```python
from build123d import *

# Parameters (mm, degrees)
SKETCH_1_R      = 1.55
SKETCH_1_W      = 22
SKETCH_1_H      = 14.8
EXTRUDE_1_DEPTH = 4
FILLET_4_R      = 3
FILLET_2_R      = 1.5


with BuildPart() as part:
    # 草图1 → 凸台-拉伸1 (new body)
    with BuildSketch(Plane.XY):
        Polygon((19, 14.5), (19, 13.5), (-18, 13.5), (-19, 13.5), (-19, -13.5), (14, -13.5), (19, -24.5), (55, -24.5), (55, 14.5), align=None)
        with BuildLine():
            ThreePointArc((-18, -9.390512484), (-18.05, -9), (-18, -8.609487516))
            ThreePointArc((-18, -8.609487516), (-14.95, -9), (-18, -9.390512484))
        make_face(mode=Mode.SUBTRACT)
        with Locations((16.5, -9)):
            Circle(SKETCH_1_R, mode=Mode.SUBTRACT)
        with BuildLine():
            ThreePointArc((31.95, -17.4), (33, -16.35), (34.05, -17.4))
            Line((34.05, -17.4), (34.05, -20.45))
            ThreePointArc((34.05, -20.45), (33, -21.5), (31.95, -20.45))
            Line((31.95, -20.45), (27.95, -20.45))
            ThreePointArc((27.95, -20.45), (26.9, -21.5), (25.85, -20.45))
            Line((25.85, -20.45), (25.85, -17.4))
            ThreePointArc((25.85, -17.4), (26.9, -16.35), (27.95, -17.4))
            Line((27.95, -17.4), (31.95, -17.4))
        make_face(mode=Mode.SUBTRACT)
        with BuildLine():
            ThreePointArc((47.95, -17.4), (49, -16.35), (50.05, -17.4))
            Line((50.05, -17.4), (50.05, -20.45))
            ThreePointArc((50.05, -20.45), (49, -21.5), (47.95, -20.45))
            Line((47.95, -20.45), (43.95, -20.45))
            ThreePointArc((43.95, -20.45), (42.9, -21.5), (41.85, -20.45))
            Line((41.85, -20.45), (41.85, -17.4))
            ThreePointArc((41.85, -17.4), (42.9, -16.35), (43.95, -17.4))
            Line((43.95, -17.4), (47.95, -17.4))
        make_face(mode=Mode.SUBTRACT)
        with Locations((22, -12.5)):
            Circle(SKETCH_1_R, mode=Mode.SUBTRACT)
        with BuildLine():
            ThreePointArc((-11.045643943, -6.5), (-11.868221008, -5.185996413), (-13, -4.126602828))
            Line((-13, -4.126602828), (-13, -1.25))
            Line((-13, -1.25), (-2, -1.25))
            Line((-2, -1.25), (-2, -6.5))
            Line((-2, -6.5), (-11.045643943, -6.5))
        make_face(mode=Mode.SUBTRACT)
        with BuildLine():
            Line((-11.045643943, 6.5), (-2, 6.5))
            Line((-2, 6.5), (-2, 1.25))
            Line((-2, 1.25), (-13, 1.25))
            Line((-13, 1.25), (-13, 4.126602828))
            ThreePointArc((-13, 4.126602828), (-11.868221008, 5.185996413), (-11.045643943, 6.5))
        make_face(mode=Mode.SUBTRACT)
        with BuildLine():
            ThreePointArc((13, -4.126602828), (11.868221008, -5.185996413), (11.045643943, -6.5))
            Line((11.045643943, -6.5), (2, -6.5))
            Line((2, -6.5), (2, -1.25))
            Line((2, -1.25), (13, -1.25))
            Line((13, -1.25), (13, -4.126602828))
        make_face(mode=Mode.SUBTRACT)
        with BuildLine():
            Line((2, 6.5), (11.045643943, 6.5))
            ThreePointArc((11.045643943, 6.5), (11.868221008, 5.185996413), (13, 4.126602828))
            Line((13, 4.126602828), (13, 1.25))
            Line((13, 1.25), (2, 1.25))
            Line((2, 1.25), (2, 6.5))
        make_face(mode=Mode.SUBTRACT)
        with BuildLine():
            ThreePointArc((-18, 8.609487516), (-18.05, 9), (-18, 9.390512484))
            ThreePointArc((-18, 9.390512484), (-14.95, 9), (-18, 8.609487516))
        make_face(mode=Mode.SUBTRACT)
        with Locations((16.5, 9)):
            Circle(SKETCH_1_R, mode=Mode.SUBTRACT)
        with Locations((22, 2.5)):
            Circle(SKETCH_1_R, mode=Mode.SUBTRACT)
        with Locations((37, -5)):
            Rectangle(SKETCH_1_W, SKETCH_1_H, mode=Mode.SUBTRACT)
        with Locations((52, -5)):
            Circle(SKETCH_1_R, mode=Mode.SUBTRACT)
        with BuildLine():
            ThreePointArc((27.95, 7.4), (26.9, 6.35), (25.85, 7.4))
            Line((25.85, 7.4), (25.85, 10.45))
            ThreePointArc((25.85, 10.45), (26.9, 11.5), (27.95, 10.45))
            Line((27.95, 10.45), (31.95, 10.45))
            ThreePointArc((31.95, 10.45), (33, 11.5), (34.05, 10.45))
            Line((34.05, 10.45), (34.05, 7.4))
            ThreePointArc((34.05, 7.4), (33, 6.35), (31.95, 7.4))
            Line((31.95, 7.4), (27.95, 7.4))
        make_face(mode=Mode.SUBTRACT)
        with BuildLine():
            ThreePointArc((43.95, 7.4), (42.9, 6.35), (41.85, 7.4))
            Line((41.85, 7.4), (41.85, 10.45))
            ThreePointArc((41.85, 10.45), (42.9, 11.5), (43.95, 10.45))
            Line((43.95, 10.45), (47.95, 10.45))
            ThreePointArc((47.95, 10.45), (49, 11.5), (50.05, 10.45))
            Line((50.05, 10.45), (50.05, 7.4))
            ThreePointArc((50.05, 7.4), (49, 6.35), (47.95, 7.4))
            Line((47.95, 7.4), (43.95, 7.4))
        make_face(mode=Mode.SUBTRACT)
    extrude(amount=EXTRUDE_1_DEPTH)

    # 圆角4
    fillet_4_edges = [part.edges().sort_by_distance(p)[0] for p in [
        (48, -12.4, 2),
        (48, 2.4, 2),
        (26, 2.4, 2),
        (26, -12.4, 2),
    ]]
    fillet(fillet_4_edges, radius=FILLET_4_R)

    # 圆角2
    # the kernel refuses this fillet: 1.5 mm, written as the material it adds along each edge
    with BuildSketch(Plane(origin=(13, -4.126602828, 0), x_dir=(-0.7799082452950566, -0.6258938639424306, 0), z_dir=(0, 0, 1)), Plane(origin=(-13, 4.126602828, 0), x_dir=(0.7799082452950533, 0.6258938639424346, 0), z_dir=(0, 0, 1))) as fillet_2_piece_1:
        with BuildLine():
            CenterArc((0.721238689, -1.49785779), FILLET_2_R, 93.062490092, 48.189685104)
            Line((-0.448623679, -0.559016994), (0, 0))
            ThreePointArc((0, 0), (0.320550528, -0.008568839), (0.641101056, 0))
        make_face()
    extrude(amount=4)
    with BuildSketch(Plane(origin=(-2, 6.5, 0), x_dir=(-1, 0, 0), z_dir=(0, 0, 1)), Plane(origin=(2, 1.25, 0), x_dir=(1, 0, 0), z_dir=(0, 0, 1)), Plane(origin=(13, 1.25, 0), x_dir=(0, 1, 0), z_dir=(0, 0, 1)), Plane(origin=(13, -1.25, 0), x_dir=(-1, 0, 0), z_dir=(0, 0, 1)), Plane(origin=(2, -1.25, 0), x_dir=(0, -1, 0), z_dir=(0, 0, 1)), Plane(origin=(2, -6.5, 0), x_dir=(1, 0, 0), z_dir=(0, 0, 1)), Plane(origin=(-2, -6.5, 0), x_dir=(0, 1, 0), z_dir=(0, 0, 1)), Plane(origin=(-2, -1.25, 0), x_dir=(-1, 0, 0), z_dir=(0, 0, 1)), Plane(origin=(-13, -1.25, 0), x_dir=(0, -1, 0), z_dir=(0, 0, 1)), Plane(origin=(-13, 1.25, 0), x_dir=(1, 0, 0), z_dir=(0, 0, 1)), Plane(origin=(-2, 1.25, 0), x_dir=(0, 1, 0), z_dir=(0, 0, 1))) as fillet_2_piece_2:
        with BuildLine():
            CenterArc((FILLET_2_R, FILLET_2_R), FILLET_2_R, 180, 90)
            Line((0, FILLET_2_R), (0, 0))
            Line((0, 0), (FILLET_2_R, 0))
        make_face()
    extrude(amount=4)
    with BuildSketch(Plane(origin=(2, 6.5, 0), x_dir=(1, 0, 0), z_dir=(0, 0, 1))) as fillet_2_piece_3:
        with BuildLine():
            CenterArc((FILLET_2_R, -FILLET_2_R), FILLET_2_R, 90, 90)
            Line((0, -FILLET_2_R), (0, 0))
            Line((0, 0), (FILLET_2_R, 0))
        make_face()
    extrude(amount=4)
    with BuildSketch(Plane(origin=(-11.045643943, 6.5, 0), x_dir=(-0.47604843493949917, -0.8794190625587175, 0), z_dir=(0, 0, 1)), Plane(origin=(11.045643943, -6.5, 0), x_dir=(0.47604843493949517, 0.8794190625587197, 0), z_dir=(0, 0, 1))) as fillet_2_piece_4:
        with BuildLine():
            CenterArc((0.895477519, 1.496696445), FILLET_2_R, 208.427635494, 57.769047364)
            Line((-0.423651075, 0.782623792), (0, 0))
            ThreePointArc((0, 0), (0.397990008, 0.013214222), (0.795980017, 0))
        make_face()
    extrude(amount=4)
    with BuildSketch(Plane(origin=(-11.045643943, -6.5, 0), x_dir=(-0.4760484349394948, 0.8794190625587198, 0), z_dir=(0, 0, 1))) as fillet_2_piece_5:
        with BuildLine():
            CenterArc((0.895477519, -1.496696445), FILLET_2_R, 93.803317142, 57.769047364)
            Line((-0.423651075, -0.782623792), (0, 0))
            ThreePointArc((0, 0), (0.397990008, -0.013214222), (0.795980017, 0))
        make_face()
    extrude(amount=4)
    with BuildSketch(Plane(origin=(-13, -4.126602828, 0), x_dir=(0.7799082452950538, -0.6258938639424342, 0), z_dir=(0, 0, 1)), Plane(origin=(13, 4.126602828, 0), x_dir=(-0.779908245295054, 0.6258938639424338, 0), z_dir=(0, 0, 1))) as fillet_2_piece_6:
        with BuildLine():
            CenterArc((0.721238689, 1.49785779), FILLET_2_R, 218.747824804, 48.189685104)
            Line((-0.448623679, 0.559016994), (0, 0))
            ThreePointArc((0, 0), (0.320550528, 0.008568839), (0.641101056, 0))
        make_face()
    extrude(amount=4)
    with BuildSketch(Plane(origin=(14, -13.5, 0), x_dir=(-1, 0, 0), z_dir=(0, 0, 1))) as fillet_2_piece_7:
        with BuildLine():
            CenterArc((FILLET_2_R * 0.643913270327, FILLET_2_R), FILLET_2_R, 204.44395478, 65.55604522)
            Line((-FILLET_2_R * 0.266453207136, FILLET_2_R * 0.586197055699), (0, 0))
            Line((0, 0), (FILLET_2_R * 0.643913270327, 0))
        make_face()
    extrude(amount=4)
    with BuildSketch(Plane(origin=(11.045643943, 6.5, 0), x_dir=(-1, 0, 0), z_dir=(0, 0, 1))) as fillet_2_piece_8:
        with BuildLine():
            CenterArc((0.889932713, 1.5), FILLET_2_R, 212.230952636, 57.769047364)
            ThreePointArc((-0.378925041, 0.7), (-0.177841682, 0.35629061), (0, 0))
            Line((0, 0), (0.889932713, 0))
        make_face()
    extrude(amount=4)
    # the kernel refuses this fillet: 1.5 mm, written as the material it takes off along each edge
    with BuildSketch(Plane(origin=(55, -24.5, -3.75), x_dir=(-1, 0, 0), z_dir=(0, 0, 1)), Plane(origin=(-19, 13.5, -3.75), x_dir=(1, 0, 0), z_dir=(0, 0, 1)), Plane(origin=(-19, -13.5, -3.75), x_dir=(0, 1, 0), z_dir=(0, 0, 1))) as fillet_2_2_piece_1:
        with BuildLine():
            CenterArc((FILLET_2_R, -FILLET_2_R), FILLET_2_R, 90, 90)
            Line((0, -FILLET_2_R), (0, 0))
            Line((0, 0), (FILLET_2_R, 0))
        make_face()
    extrude(amount=11.5, mode=Mode.SUBTRACT)
    with BuildSketch(Plane(origin=(55, 14.5, -3.75), x_dir=(-1, 0, 0), z_dir=(0, 0, 1))) as fillet_2_2_piece_2:
        with BuildLine():
            CenterArc((FILLET_2_R, FILLET_2_R), FILLET_2_R, 180, 90)
            Line((0, FILLET_2_R), (0, 0))
            Line((0, 0), (FILLET_2_R, 0))
        make_face()
    extrude(amount=11.5, mode=Mode.SUBTRACT)
    with BuildSketch(Plane(origin=(19, 14.5, -3.535533906), x_dir=(1, 0, 0), z_dir=(0, 0, 1))) as fillet_2_2_piece_3:
        with BuildLine():
            CenterArc((1.414213562, -1.5), FILLET_2_R, 90, 70.528779366)
            Line((0, -1), (0, 0))
            Line((0, 0), (1.414213562, 0))
        make_face()
    extrude(amount=11.071067812, mode=Mode.SUBTRACT)
    with BuildSketch(Plane(origin=(19, -24.5, -2.414674764), x_dir=(-0.4138029443011837, 0.9103664774626049, 0), z_dir=(0, 0, 1))) as fillet_2_2_piece_4:
        with BuildLine():
            CenterArc((FILLET_2_R * 0.643913270327, -FILLET_2_R), FILLET_2_R, 90, 65.55604522)
            Line((-FILLET_2_R * 0.266453207136, -FILLET_2_R * 0.586197055699), (0, 0))
            Line((0, 0), (FILLET_2_R * 0.643913270327, 0))
        make_face()
    extrude(amount=8.829349527, mode=Mode.SUBTRACT)


solid = part.part
```
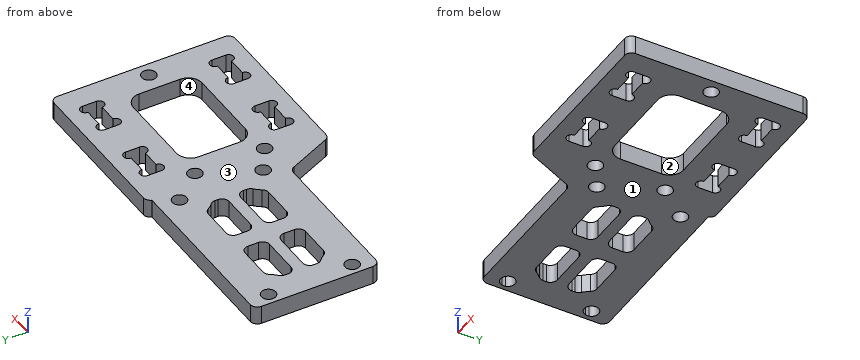
Geometry check sheet. Reference: the model listing, model coordinates, mm. Face numbers are marked on the shaded views. A direction names the side the tool comes from. Coordinates: 2 decimals unless noted, no trailing zeros. Order: outer loops, then holes, each group sorted by start corner. A loop starts at its lowest first (then second) coordinate and runs counter-clockwise, first axis right, second up. Notation, with made-up numbers: M 79.25,-19.5 L 96.25,-19.5 A12 cw 96.25,-6.5 Z; hole C 31,1.5 d10. An arc over 180 degrees is marked long. Answer as a JSON object with one key per item and string values.
Q1. Cross-section at B-B on x = -5. Record the cut outline in (y, z).
Results are:
{"outline": "M -13.5,0 L -6.5,0 L -6.5,4 L -13.5,4 Z; M -1.25,0 L 1.25,0 L 1.25,4 L -1.25,4 Z; M 6.5,0 L 13.5,0 L 13.5,4 L 6.5,4 Z"}
Q2. Release check for a two-part mould opening along X. For the marked faces 1 and 2 record: released by +X, released by -X, zero draft, split by the parting line, or undercut.
Results are:
{"face 1": "zero draft", "face 2": "undercut"}
Q3. Cross-section at D-D on z = 3.3. Give the number of separate pieces and of enclosed holes in the cut face, and give its area (3 significant figures).
Results are:
{"separate pieces": "1", "enclosed holes": "16", "area": "1,740 mm²"}
Q4. Cross-section at A-A on x = 52. Record the cut outline in (y, z), and give its area (3 significant figures).
Results are:
{"outline": "M -24.5,0 L -6.55,0 L -6.55,4 L -24.5,4 Z; M -3.45,0 L 14.5,0 L 14.5,4 L -3.45,4 Z", "area": "144 mm²"}
Q5. Cross-section at C-C on x = 33. Record the cut outline in (y, z), and give its area (3 significant figures).
Results are:
{"outline": "M -24.5,0 L -21.5,0 L -21.5,4 L -24.5,4 Z; M -16.35,0 L -12.4,0 L -12.4,4 L -16.35,4 Z; M 2.4,0 L 6.35,0 L 6.35,4 L 2.4,4 Z; M 11.5,0 L 14.5,0 L 14.5,4 L 11.5,4 Z", "area": "55.6 mm²"}
Q6. Tool access check on the marked faces 3 and 4. Record the directions out of +Z, -Z, +X, -X, +Y, -Y that give a thin tool (end or side, any length) a straight path to the whole face; none if there is none.
Results are:
{"face 3": "+Z, +X, -X, +Y, -Y", "face 4": "+Z, -Z"}
Q7. Scan lines: line 1 (Y direction, x = 6.5, z = 0.75); line 2 (Y direction, x = 22, z = 3); line 3 (Y direction, x = 46, z = 2.3). Record each from-to range of solid material in increasing order.
Results are:
{"line 1": "y = -13.5 to -6.5, -1.25 to 1.25, 6.5 to 13.5", "line 2": "y = -24.5 to -14.05, -10.95 to 0.95, 4.05 to 14.5", "line 3": "y = -24.5 to -20.45, -17.4 to -12.23, 2.23 to 7.4, 10.45 to 14.5"}
Q8. Depth check by flat-ended pin: pin 1 Ø1.2 at (x, z) = (9, 2.5) entering from +Y; pin 2 Ø0.9 at (y, z) = (-19.5, 2.5) entering from -X; pin 3 Ø3 at (x, y) = (22, -12.5) entering from -Z; pin 4 Ø1.2 at (x, z) = (-7, 2.5) entering from -Y. Enter the tip coordinate at first touch or a pass-through.
Results are:
{"pin 1": "stops at y = 13.5", "pin 2": "stops at x = 16.52", "pin 3": "passes through", "pin 4": "stops at y = -13.5"}
